Autodesk Fusion 360 part; units mm, degrees
sketch "Sketch1" plane through (0, 0, 0) normal (0, 0, 1) x (1, 0, 0)
  line L0 (0, 0) -> (-10, 0)
  line L1 (-10, 0) -> (-10, -26)
  line L2 (-10, -26) -> (0, -26)
  line L3 (0, -26) -> (0, 0)
  dimension "d1" = 10
  dimension "d2" = 26
extrude "Extrude1" add sketch "Sketch1" along normal blind 2
sketch "Sketch2" plane through (0, 0, 2) normal (0, 0, 1) x (-1, 0, 0)
  line L0 (0, 26) -> (0, 0)
  line L1 (0, 0) -> (10, 0)
  line L2 (10, 0) -> (10, 26)
  line L3 (10, 26) -> (0, 26)
  circle A0 centre (5, 21) radius 1
  circle A1 centre (5, 7.0039) radius 1
  point P0 (4.5847, 3.0102)
  dimension "d5" = 2
  dimension "d6" = 2
  dimension "d8" = 5
  dimension "d9" = 5
  dimension "d10" = 13.9961
  dimension "d11" = 5
extrude "Extrude2" cut sketch "Sketch2" against normal blind 10 contours A0 | A1
chamfer "Chamfer1" distance 1.5 angle 45 4 edges at (-5, -26, 2) (0, -13, 2) (-10, -13, 2) (-5, 0, 2) measured on face at (-5.0249, -2.0022, 2) measured on face at (-5.0249, -2.0022, 2) measured on face at (-5.0249, -2.0022, 2) measured on face at (-5.0249, -2.0022, 2)
The model under review builds one solid part; all positions refer to its coordinate system, in mm. Give positions to 0.01 mm unless a question says otherwise; leave off trailing zeros. Write each loop counter-clockwise with the first axis right and the second up, starting at its lowest first coordinate (ties: lowest second). Pieces come first, ordered by that corner, then holes.
1. Draft analysis for pull direction X (two halves, no side actions). For faces 1 (the cylindrical face through (-4.206, -6.395, 1.014)), 2 (the flat face through (-9.3, -12.8, 1.2)), 3 (the cylindrical face through (-5, -20, 1)), 4 (the flat face through (-5, -13, 0)), state which applies: +X half, -X half, draft (parallel to the pull), parting line (faces both ways), or undercut.
2. Add section B-B, the plane y = -21. Write out the cut boundary in (x, z).
3. For P1, Ø1.8, axis at x = -5, y = -7, coming from the -Z side, flat-tipped, find the tip position at first contact; note if it passes through.
4. Add section C-C, the plane x = -8. Write out the cut boundary in (y, z), plus the area to 4 significant figures.
5. Wall thickness on L1, parallel to Y at x = -5, z = 0.4; L2, parallel to Y at x = -5, z = 1; L3, parallel to X at y = -20.25, z = 1.5: over which ranges is each line inside the solid? List them lowest first.
6. Add section D-D, the plane z = 1.25. Write out the cut boundary in (x, y).
7. Add section A-A, the plane x = -5. Write out the cut boundary in (y, z).
Worked answers:
1. face 1: undercut
1. face 2: -X half
1. face 3: undercut
1. face 4: draft
2. outline: (-10, 0) - (-6, 0) - (-6, 2) - (-8.5, 2) - (-10, 0.5) - close; (-4, 0) - (0, 0) - (0, 0.5) - (-1.5, 2) - (-4, 2) - close
3. P1: passes through
4. outline: (-26, 0) - (0, 0) - (0, 0.5) - (-1.5, 2) - (-24.5, 2) - (-26, 0.5) - close
4. area: 49.75 mm2
5. L1: y = -26 to -22, -20 to -8, -6 to 0
5. L2: y = -25.5 to -22, -20 to -8, -6 to -0.5
5. L3: x = -9 to -5.66, -4.34 to -1
6. outline: (-9.25, -25.25) - (-0.75, -25.25) - (-0.75, -0.75) - (-9.25, -0.75) - close; hole circle Ø2 at (-5, -21); hole circle Ø2 at (-5, -7)
7. outline: (-26, 0) - (-22, 0) - (-22, 2) - (-24.5, 2) - (-26, 0.5) - close; (-20, 0) - (-8, 0) - (-8, 2) - (-20, 2) - close; (-6, 0) - (0, 0) - (0, 0.5) - (-1.5, 2) - (-6, 2) - close
